Source: CAD feature listing. Evaluate the final solid. Frame: model axes, mm. A direction names the side the tool comes from. Give positions to 0.01 mm unless a question says otherwise; leave off trailing zeros. Order: outer loops, then holes, each group sorted by start corner. A loop starts at its lowest first (then second) coordinate and runs counter-clockwise, first axis right, second up.
```python
from build123d import *

# Parameters (mm, degrees)
SKETCH_3_R                   = 25
EXTRUDE_1_DEPTH              = 2
SKETCH_4_R                   = 25
SKETCH_4_R_2                 = 17.5
EXTRUDE_2_DEPTH              = 1
SKETCH_5_R                   = 25
SKETCH_5_R_2                 = 18.5
EXTRUDE_3_DEPTH              = 7
SKETCH_6_R                   = 25
SKETCH_6_R_2                 = 17.5
EXTRUDE_4_DEPTH              = 2
EXTRUDE_5_DEPTH              = 9
SKETCH_11_R                  = 8.5
CUT_EXTRUDE_3_DEPTH          = 111
SKETCH_12_R                  = 9.5
CUT_EXTRUDE_4_DEPTH          = 2.5
SKETCH_13_R                  = 9.5
EXTRUDE_6_DEPTH              = 5
HOLE_WIZARD_M4_1_D           = 4.5
HOLE_WIZARD_M4_1_CBORE_D     = 8
HOLE_WIZARD_M4_1_CBORE_DEPTH = 4.4
PATTERN_CIRCULAR_1_COUNT     = 3
SKETCH_17_W                  = 17.714059585
SKETCH_17_H                  = 64.604217311
CUT_EXTRUDE_5_DEPTH          = 1111


with BuildPart() as part:
    # 스케치3 → 보스-돌출1 (new body)
    with BuildSketch(Plane(origin=(0, 0, 0), x_dir=(0, 0, -1), z_dir=(1, 0, 0))):
        Circle(SKETCH_3_R)
    extrude(amount=EXTRUDE_1_DEPTH)

    # 스케치4 → 보스-돌출2 (add)
    with BuildSketch(Plane(origin=(2, 0, 0), x_dir=(0, 0, -1), z_dir=(1, 0, 0))):
        Circle(SKETCH_4_R)
        Circle(SKETCH_4_R_2, mode=Mode.SUBTRACT)
    extrude(amount=EXTRUDE_2_DEPTH)

    # 스케치5 → 보스-돌출3 (add)
    with BuildSketch(Plane(origin=(3, 0, 0), x_dir=(0, 0, -1), z_dir=(1, 0, 0))):
        Circle(SKETCH_5_R)
        Circle(SKETCH_5_R_2, mode=Mode.SUBTRACT)
    extrude(amount=EXTRUDE_3_DEPTH)

    # 스케치6 → 보스-돌출4 (add)
    with BuildSketch(Plane(origin=(10, 0, 0), x_dir=(0, 0, -1), z_dir=(1, 0, 0))):
        Circle(SKETCH_6_R)
        Circle(SKETCH_6_R_2, mode=Mode.SUBTRACT)
    extrude(amount=EXTRUDE_4_DEPTH)

    # 스케치10 → 보스-돌출5 (add)
    with BuildSketch(Plane(origin=(12, 0, 0), x_dir=(0, 0, -1), z_dir=(1, 0, 0))):
        with BuildLine():
            Line((4.166666667, 24.65033243), (62.5, 14.790199458))
            ThreePointArc((62.5, 14.790199458), (75, 0), (62.5, -14.790199458))
            Line((62.5, -14.790199458), (4.166666667, -24.65033243))
            ThreePointArc((4.166666667, -24.65033243), (25, 0), (4.166666667, 24.65033243))
        make_face()
    extrude(amount=-EXTRUDE_5_DEPTH)

    # 스케치11 → 컷-돌출3 (cut, symmetric)
    with BuildSketch(Plane(origin=(7.5, 0, 0), x_dir=(0, 0, -1), z_dir=(1, 0, 0))):
        with Locations((60, 0)):
            Circle(SKETCH_11_R)
    extrude(amount=CUT_EXTRUDE_3_DEPTH, both=True, mode=Mode.SUBTRACT)

    # 스케치12 → 컷-돌출4 (cut, symmetric)
    with BuildSketch(Plane(origin=(7.5, 0, 0), x_dir=(0, 0, -1), z_dir=(1, 0, 0))):
        with Locations((60, 0)):
            Circle(SKETCH_12_R)
    extrude(amount=CUT_EXTRUDE_4_DEPTH, both=True, mode=Mode.SUBTRACT)

    # 스케치13 → 보스-돌출6 (add)
    with BuildSketch(Plane.ZY):
        Circle(SKETCH_13_R)
    extrude(amount=EXTRUDE_6_DEPTH)

    # M4 육각 소켓 머리 캡 나사용 카운터보어1 (through all)
    with Locations(Plane(origin=(2, 0, 0), x_dir=(0, 0, -1), z_dir=(1, 0, 0))):
        with Locations((0, 5)):
            hole_wizard_m4_1 = CounterBoreHole(HOLE_WIZARD_M4_1_D / 2, HOLE_WIZARD_M4_1_CBORE_D / 2, HOLE_WIZARD_M4_1_CBORE_DEPTH)

    # 원형 패턴1: M4 육각 소켓 머리 캡 나사용 카운터보어1 ×3 about axis
    pattern_circular_1_axis = Axis((0, 0, 0), (1, 0, 0))
    for i in range(1, PATTERN_CIRCULAR_1_COUNT):
        add(hole_wizard_m4_1.rotate(pattern_circular_1_axis, i * 360 / PATTERN_CIRCULAR_1_COUNT), mode=Mode.SUBTRACT)

    # 스케치17 → 컷-돌출5 (cut, symmetric)
    with BuildSketch(Plane.XY):
        with Locations((15.857029793, -1.852450676)):
            Rectangle(SKETCH_17_W, SKETCH_17_H)
    extrude(amount=CUT_EXTRUDE_5_DEPTH, both=True, mode=Mode.SUBTRACT)


solid = part.part
```
1) Section query B-B, the plane y = -2.5. Count the separate pieces of the cut face and the enclosed holes in it, and give its area (3 significant figures).
Report:
separate pieces: 4
enclosed holes: 0
area: 295 mm2
2) Material intervals for L1, parallel to Z at x = 0.25, y = -1; L2, parallel to Y at x = -1.5, z = -1.5; L3, parallel to X at y = -12, z = -50, sorted ascending.
Report:
L1: z = -24.98 to -8.04, -0.62 to 0.62, 8.04 to 24.98
L2: y = -9.38 to -5.33, 0.33 to 1.29, 8.71 to 9.38
L3: x = 3 to 7
3) Draft query along Y for faces 1 (the cylindrical face through (5, 0, -75)), 2 (the flat face through (-5, 0, 0)), 3 (the cylindrical face through (4.01, 0.37, -51.51)). Return one class per face: +Y half, -Y half, draft (parallel to the pull), parting line (faces both ways), or undercut.
Report:
face 1: parting line
face 2: draft
face 3: undercut
4) Section query D-D, the plane y = 20. Return the cut outline in (x, z).
Report:
outline: (0, -15) - (3, -15) - (3, -31.68) - (7, -31.68) - (7, 15) - (0, 15) - close
5) Reachability of faces 4 (the flat face through (3, -14, 11)), 5 (the flat face through (7, 0, -24)), 6 (the cylindrical face through (-2.46, -8.43, 4.38)) from +Z, -Z, +X, -X, +Y, -Y: full face, straight path, thin tool, end or side. Return the list, or none.
Report:
face 4: +X
face 5: +Z, -Z, +X, +Y, -Y
face 6: -X
6) Pin query (flat end, axial travel): pin 1 (2 mm diameter, centred on x = -0.5, y = -3, fed in from +Z); pin 2 (5 mm diameter, centred on y = -2.5, z = -4.33, fed in from +X); pin 3 (6 mm diameter, centred on x = 0, y = -9.5, fed in from +Z). Return the tip coordinate at first contact, or that it passes through.
Report:
pin 1: stops at z = 24.91
pin 2: stops at x = -2.4
pin 3: stops at z = 24.14
7) Section query A-A, the plane z = -60. Return the cut outline in (x, y), and give its area (3 significant figures).
Report:
outline: (3, -15.21) - (7, -15.21) - (7, -9.5) - (5, -9.5) - (5, -8.5) - (3, -8.5) - close; (3, 8.5) - (5, 8.5) - (5, 9.5) - (7, 9.5) - (7, 15.21) - (3, 15.21) - close
area: 49.7 mm2
8) Section query C-C, the plane z = -11.5. Return the cut outline in (x, y), and give its area (3 significant figures).
Report:
outline: (0, -22.2) - (3, -22.2) - (3, -23.41) - (7, -23.41) - (7, -14.49) - (3, -14.49) - (3, -13.19) - (2, -13.19) - (2, 13.19) - (3, 13.19) - (3, 14.49) - (7, 14.49) - (7, 23.41) - (3, 23.41) - (3, 22.2) - (0, 22.2) - close
area: 178 mm2
